Geometry check sheet. Reference: the model listing, model coordinates, mm. A direction names the side the tool comes from. Round coordinates to 2 decimals unless told otherwise and drop trailing zeros. Write each loop counter-clockwise with the first axis right and the second up, starting at its lowest first coordinate (ties: lowest second). Pieces come first, ordered by that corner, then holes. Notation, with made-up numbers: (30.25, 9.5) -> (47.25, 9.5) arc R25 cw to (47.25, 37.5) -> close; hole circle Ø4 at (74.5, -29.5). An arc over 180 degrees is marked (long way). Use a Markdown table: item, result.
```python
from build123d import *

# Parameters (mm, degrees)
F0_W     = 19.05
F0_H     = 33.02
F1_DEPTH = 19.05
F2_DEPTH = 6.35
F3_DEPTH = 6.35


with BuildPart() as f1:
    # F0 (on Right) → F1 (new body)
    with BuildSketch(Plane.YZ):
        Polygon((-570.548746, 72.287804), (-583.248746, 72.287804), (-583.248746, 39.267804), (-564.198746, 39.267804), (-564.198746, 6.247804), (-564.198746, -26.772196), (-564.198746, -59.792196), (-564.198746, -80.112196), (147.001254, -80.112196), (147.001254, -59.792196), (147.001254, -26.772196), (147.001254, -10.262196), (147.001254, 6.247804), (147.001254, 39.267804), (147.001254, 59.587804), (-564.198746, 59.587804), (-570.548746, 59.587804), align=None)
        Polygon((-564.198746, 72.287804), (-570.548746, 72.287804), (-570.548746, 59.587804), (-564.198746, 59.587804), (147.001254, 59.587804), (153.351254, 59.587804), (153.351254, 72.287804), (147.001254, 72.287804), align=None)
        with Locations((-573.723746, -10.262196)):
            Rectangle(F0_W, F0_H)
        Polygon((166.051254, 72.287804), (153.351254, 72.287804), (153.351254, 59.587804), (147.001254, 59.587804), (147.001254, 39.267804), (166.051254, 39.267804), align=None)
        Polygon((-564.198746, -80.112196), (-564.198746, -59.792196), (-583.248746, -59.792196), (-583.248746, -92.812196), (-570.548746, -92.812196), (-570.548746, -80.112196), align=None)
        Polygon((166.051254, 6.247804), (147.001254, 6.247804), (147.001254, -10.262196), (147.001254, -26.772196), (166.051254, -26.772196), align=None)
        Polygon((147.001254, -80.112196), (-564.198746, -80.112196), (-570.548746, -80.112196), (-570.548746, -92.812196), (-564.198746, -92.812196), (147.001254, -92.812196), (153.351254, -92.812196), (153.351254, -80.112196), align=None)
        Polygon((147.001254, -59.792196), (147.001254, -80.112196), (153.351254, -80.112196), (153.351254, -92.812196), (166.051254, -92.812196), (166.051254, -59.792196), align=None)
    extrude(amount=F1_DEPTH)

    # F0 (on Right) → F2 (cut)
    with BuildSketch(Plane.YZ):
        Polygon((-564.198746, 72.287804), (-570.548746, 72.287804), (-570.548746, 59.587804), (-564.198746, 59.587804), (147.001254, 59.587804), (153.351254, 59.587804), (153.351254, 72.287804), (147.001254, 72.287804), align=None)
    extrude(amount=F2_DEPTH, mode=Mode.SUBTRACT)

    # F0 (on Right) → F3 (cut)
    with BuildSketch(Plane.YZ):
        Polygon((147.001254, -80.112196), (-564.198746, -80.112196), (-570.548746, -80.112196), (-570.548746, -92.812196), (-564.198746, -92.812196), (147.001254, -92.812196), (153.351254, -92.812196), (153.351254, -80.112196), align=None)
    extrude(amount=F3_DEPTH, mode=Mode.SUBTRACT)


solid = f1.part
```
(1) Gauge pin test, flat ends, axial feed: pin 1 Ø5 at (x, y) = (4, -344) entering from +Z; pin 2 Ø6.5 at (y, z) = (-282, -85.5) entering from -X; pin 3 Ø1.9 at (x, y) = (2, -254.5) entering from -Z; pin 4 Ø10 at (x, z) = (12.5, 16) entering from +Y. Record the tip position at first contact, or that the pin passes through.
A:
| item | result |
|---|---|
| pin 1 | stops at z = 72.29 |
| pin 2 | stops at x = 6.35 |
| pin 3 | stops at z = -80.11 |
| pin 4 | stops at y = 147 |
(2) Access from +Z, -Z, +X, -X, +Y, -Y to the whole of each face (thin tool, end or side, straight path). Record for faces 1 (the face through (9, 156, 39.268)), 2 (the face through (6.35, -214, 66)), 3 (the face through (9, -564.199, 23)).
A:
| item | result |
|---|---|
| face 1 | +X, -X, +Y |
| face 2 | +Z, -X |
| face 3 | +X, -X, -Y |
(3) Section check C-C on z = -43. Record the cut outline in (x, y).
A:
| item | result |
|---|---|
| outline | (0, -564.2) -> (19.05, -564.2) -> (19.05, 147) -> (0, 147) -> close |
(4) Section check A-A on x = 10.25. Record the cut outline in (y, z).
A:
| item | result |
|---|---|
| outline | (-583.25, -92.81) -> (166.05, -92.81) -> (166.05, -59.79) -> (147, -59.79) -> (147, -26.77) -> (166.05, -26.77) -> (166.05, 6.25) -> (147, 6.25) -> (147, 39.27) -> (166.05, 39.27) -> (166.05, 72.29) -> (-583.25, 72.29) -> (-583.25, 39.27) -> (-564.2, 39.27) -> (-564.2, 6.25) -> (-583.25, 6.25) -> (-583.25, -26.77) -> (-564.2, -26.77) -> (-564.2, -59.79) -> (-583.25, -59.79) -> close |
(5) Section check B-B on y = 55.5. Record the cut outline in (x, z), plus the area to 3 significant figures.
A:
| item | result |
|---|---|
| outline | (0, -80.11) -> (6.35, -80.11) -> (6.35, -92.81) -> (19.05, -92.81) -> (19.05, 72.29) -> (6.35, 72.29) -> (6.35, 59.59) -> (0, 59.59) -> close |
| area | 2,980 mm2 |
(6) Release check for a two-part mould opening along Z. For faces 4 (the face through (14, -214, -92.812)), 5 (the face through (9, -583.249, -10)), 6 (the face through (9, 157, 6.248)) record: +Z half, -Z half, draft (parallel to the pull), parting line (faces both ways), or undercut.
A:
| item | result |
|---|---|
| face 4 | -Z half |
| face 5 | draft |
| face 6 | undercut |
(7) Thickness scan on line 1 (Y direction, x = 5.5, z = 62); line 2 (Z direction, x = 1.75, y = -343.5); line 3 (X direction, y = -108.5, z = -81). Record the ranges inside material, lowest first.
A:
| item | result |
|---|---|
| line 1 | y = -583.25 to -570.55, 153.35 to 166.05 |
| line 2 | z = -80.11 to 59.59 |
| line 3 | x = 6.35 to 19.05 |
